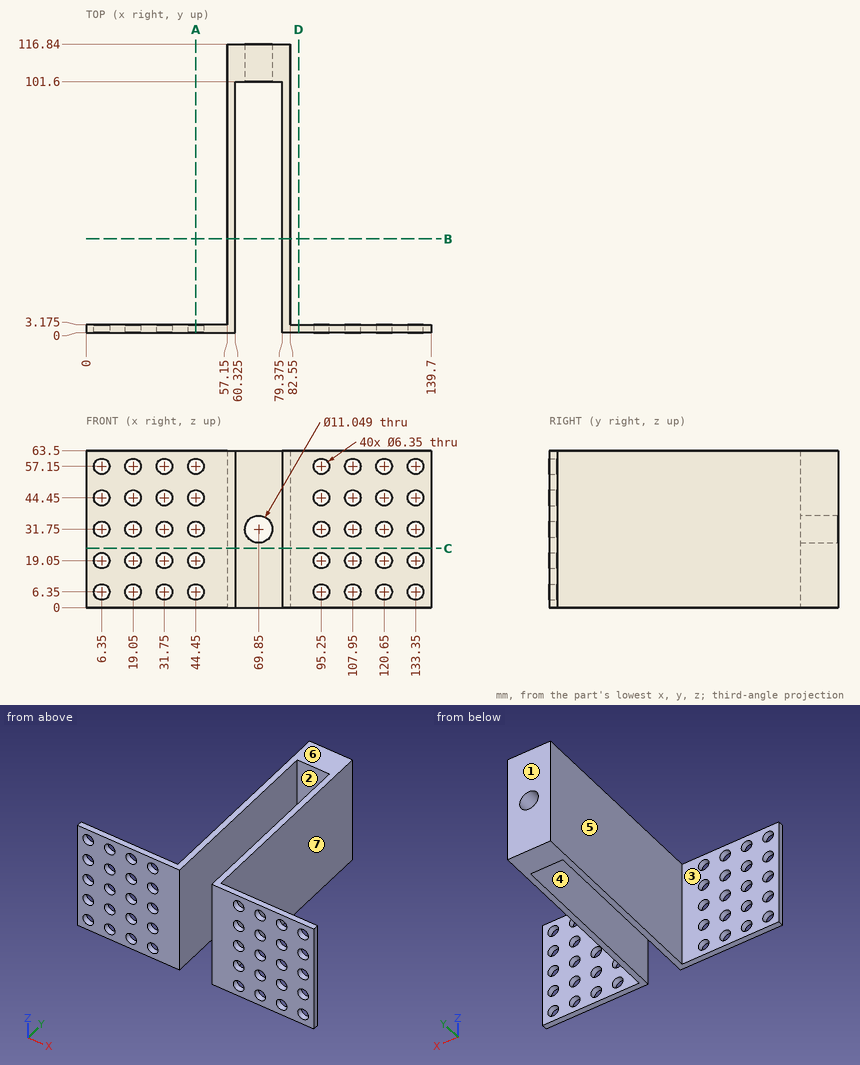
Answer from the drawing. Dimensions are ordinates in mm from the lowest x, y and z of the part. A direction names the side the tool comes from. Coordinates: 2 decimals unless noted, no trailing zeros. Loops run counter-clockwise (first coordinate to the right, second up) from the corner with the lowest first, then second, coordinate; pieces in that order, holes last. Notation, with made-up numbers: (60.25, 44) - (86.25, 44) arc R19 ccw to (86.25, 51) - close; hole circle Ø2 at (6.5, -32). An arc over 180 degrees is marked (long way). Use a Markdown table: item, result.
Item 1: Consider probe 1 along Z at (x, y) = (31.75, 1.45) (3 decimals); probe 2 along X at (y, z) = (9, 26) (3 decimals); probe 3 along Y at (x, z) = (79, 16). Determine where each line is inside the solid, lowest interval first. Write a range as from..to.
Evaluation:
| item | result |
|---|---|
| probe 1 | z = 0..3.175, 9.525..15.875, 22.225..28.575, 34.925..41.275, 47.625..53.975, 60.325..63.5 |
| probe 2 | x = 57.15..60.325, 79.375..82.55 |
| probe 3 | y = 101.6..116.84 |
Item 2: Find section C-C, the plane z = 24. Determine the outline of the cut face in (x, y) (3 decimals), and give its area (3 significant figures).
Evaluation:
| item | result |
|---|---|
| outline | (0, 0) - (60.325, 0) - (60.325, 101.6) - (79.375, 101.6) - (79.375, 0) - (139.7, 0) - (139.7, 3.175) - (82.55, 3.175) - (82.55, 116.84) - (57.15, 116.84) - (57.15, 3.175) - (0, 3.175) - close |
| area | 1,400 mm2 |
Item 3: The mould has two halves that part along X. Classify the marked faces 4, 5, 6 and 7: +X half, -X half, draft (parallel to the pull), parting line (faces both ways), or undercut.
Evaluation:
| item | result |
|---|---|
| face 4 | undercut |
| face 5 | -X half |
| face 6 | draft |
| face 7 | +X half |
Item 4: Find section D-D, the plane x = 86. Determine the outline of the cut face in (y, z) (3 decimals).
Evaluation:
| item | result |
|---|---|
| outline | (0, 0) - (3.175, 0) - (3.175, 63.5) - (0, 63.5) - close |
Item 5: For the marked faces 1, 2 and 3, determine the directions among +Z, -Z, +X, -X, +Y, -Y from which every point of the face is accessible in a straight line to the end or side of a thin tool.
Evaluation:
| item | result |
|---|---|
| face 1 | +Z, -Z, +X, -X, +Y |
| face 2 | +Z, -Z, -Y |
| face 3 | +Z, -Z, -X, +Y |
Item 6: Find section B-B, the plane y = 38. Determine the outline of the cut face in (x, z) (3 decimals).
Evaluation:
| item | result |
|---|---|
| outline | (57.15, 0) - (60.325, 0) - (60.325, 63.5) - (57.15, 63.5) - close; (79.375, 0) - (82.55, 0) - (82.55, 63.5) - (79.375, 63.5) - close |
Item 7: Given pin 1 Ø7.5 at (x, z) = (133.35, 57.15) entering from +Y (3 decimals); pin 2 Ø12 at (y, z) = (19.5, 44) entering from -X; pin 3 Ø10 at (y, z) = (41, 10) entering from +X; pin 4 Ø5 at (x, z) = (19.05, 44.45) entering from -Y, each flat-ended and moving along its own axis, determine where each tip first touches the part or whether it passes through.
Evaluation:
| item | result |
|---|---|
| pin 1 | stops at y = 3.175 |
| pin 2 | stops at x = 57.15 |
| pin 3 | stops at x = 82.55 |
| pin 4 | passes through |
Item 8: Find section A-A, the plane x = 44.45. Determine the outline of the cut face in (y, z) (3 decimals), and give its area (3 significant figures).
Evaluation:
| item | result |
|---|---|
| outline | (0, 0) - (3.175, 0) - (3.175, 3.175) - (0, 3.175) - close; (0, 9.525) - (3.175, 9.525) - (3.175, 15.875) - (0, 15.875) - close; (0, 22.225) - (3.175, 22.225) - (3.175, 28.575) - (0, 28.575) - close; (0, 34.925) - (3.175, 34.925) - (3.175, 41.275) - (0, 41.275) - close; (0, 47.625) - (3.175, 47.625) - (3.175, 53.975) - (0, 53.975) - close; (0, 60.325) - (3.175, 60.325) - (3.175, 63.5) - (0, 63.5) - close |
| area | 101 mm2 |
